Verification items for the finished model (mm, model axes). A direction names the side the tool comes from. Give positions to 0.01 mm unless a question says otherwise; leave off trailing zeros. Loops run counter-clockwise (first coordinate to the right, second up) from the corner with the lowest first, then second, coordinate; pieces in that order, holes last. Notation, with made-up numbers: (61.25, -5.5) -> (69.25, -5.5) arc R19 ccw to (69.25, 12.5) -> close; hole circle Ø8 at (77.25, -15.75). An arc over 180 degrees is marked (long way). Answer in a Markdown table with one row per item. Add a question column.
Q1. Section check A-A on x = 0. Enter the section's corners in (y, z) (3 decimals).
Q2. Section check B-B on z = 2.6. Enter the section's corners in (x, y) (3 decimals).
Q3. Material ranges on probe 1 along Z at (x, y) = (2.25, 0.25); probe 2 along X at (y, z) = (0, 0.1) (3 decimals); probe 3 along Y at (x, z) = (-0.25, 2.4) (3 decimals), recorded low to high.
Q4. Section check D-D on y = 1.5. Enter the section's corners in (x, z), and give its area (3 significant figures).
Q5. Set-up check for faces 1 (the face through (0, 2.625, 2)), 2 (the face through (2, -4.625, 1)), 3 (the face through (3.897, -2, 1)), 4 (the face through (-1, -5, 1)), 5 (the face through (0, 3.625, 1)): record each of +Z, -Z, +X, -X, +Y, -Y from which the full face is reachable in a straight line by a thin tool's end or side.
Q6. Gauge pin test, flat ends, axial feed: P1, Ø0.9, axis at x = 2, z = 2, coming from the -Y side (3 decimals); P2, Ø2.5, axis at x = 0, y = 0, coming from the +Z side; P3, Ø0.8, axis at y = -5.5, z = 1.5, coming from the +X side; P4, Ø3.5, axis at x = 0, y = 0, coming from the +Z side. Record the tip position at first contact, or that the pin passes through.
Q7. Section check C-C on y = -0.5. Enter the section's corners in (x, z), and give its area (3 significant figures).
Q8. Release check for a two-part mould opening along Z. For faces 6 (the face through (-0.3, -1.34, 0.26)), 7 (the face through (2.284, 1.294, 1.514)), 8 (the face through (-2.263, 1.331, 1.514)), 9 (the face through (0, -2, 0)) record: pulls with the +Z half, pulls with the -Z half, needs draft (parallel to the pull), parting line crosses it, or undercut.
```python
from build123d import *

# Parameters (mm, degrees)
SKETCH1_R           = 1.375
BOSS_EXTRUDE1_DEPTH = 3
CUT_EXTRUDE1_DEPTH  = 0.98


with BuildPart() as part:
    # Sketch1 → Boss-Extrude1 (new body)
    with BuildSketch(Plane.XY):
        Polygon((-1, -4.625), (-1, -6.125), (1, -6.125), (1, -4.625), (3.897114317, -4.625), (3.897114317, 0.5), (2.092894726, 3.625), (-2.092894726, 3.625), (-3.897114317, 0.5), (-3.897114317, -4.625), align=None)
        Circle(SKETCH1_R, mode=Mode.SUBTRACT)
    extrude(amount=BOSS_EXTRUDE1_DEPTH)

    # Sketch2 → Cut-Extrude1 (cut, symmetric)
    with BuildSketch(Plane.XY.offset(1.5)):
        Polygon((-1.515544457, -2.625), (1.515544457, -2.625), (3.031088913, 0), (1.515544457, 2.625), (-1.515544457, 2.625), (-3.031088913, 0), align=None)
    extrude(amount=CUT_EXTRUDE1_DEPTH, both=True, mode=Mode.SUBTRACT)


solid = part.part
```
Taken from the geometry:
| question | item | result |
|---|---|---|
| 1 | outline | (-6.125, 0) -> (-1.375, 0) -> (-1.375, 0.52) -> (-2.625, 0.52) -> (-2.625, 2.48) -> (-1.375, 2.48) -> (-1.375, 3) -> (-6.125, 3) -> close; (1.375, 0) -> (3.625, 0) -> (3.625, 3) -> (1.375, 3) -> (1.375, 2.48) -> (2.625, 2.48) -> (2.625, 0.52) -> (1.375, 0.52) -> close |
| 2 | outline | (-3.897, -4.625) -> (-1, -4.625) -> (-1, -6.125) -> (1, -6.125) -> (1, -4.625) -> (3.897, -4.625) -> (3.897, 0.5) -> (2.093, 3.625) -> (-2.093, 3.625) -> (-3.897, 0.5) -> close; hole circle Ø2.75 at (0, 0) |
| 3 | probe 1 | z = 0 to 0.52, 2.48 to 3 |
| 3 | probe 2 | x = -3.897 to -1.375, 1.375 to 3.897 |
| 3 | probe 3 | y = -6.125 to -2.625, 2.625 to 3.625 |
| 4 | outline | (-3.32, 0) -> (3.32, 0) -> (3.32, 3) -> (-3.32, 3) -> close; hole (-2.17, 0.52) -> (2.17, 0.52) -> (2.17, 2.48) -> (-2.17, 2.48) -> close |
| 4 | area | 11.4 mm² |
| 5 | face 1 | none |
| 5 | face 2 | +Z, -Z, +X, -Y |
| 5 | face 3 | +Z, -Z, +X, +Y, -Y |
| 5 | face 4 | +Z, -Z, -X, -Y |
| 5 | face 5 | +Z, -Z, +X, -X, +Y |
| 6 | P1 | stops at y = -4.625 |
| 6 | P2 | passes through |
| 6 | P3 | stops at x = 1 |
| 6 | P4 | stops at z = 3 |
| 7 | outline | (-3.9, 0) -> (-1.28, 0) -> (-1.28, 0.52) -> (-2.74, 0.52) -> (-2.74, 2.48) -> (-1.28, 2.48) -> (-1.28, 3) -> (-3.9, 3) -> close; (1.28, 0) -> (3.9, 0) -> (3.9, 3) -> (1.28, 3) -> (1.28, 2.48) -> (2.74, 2.48) -> (2.74, 0.52) -> (1.28, 0.52) -> close |
| 7 | area | 9.97 mm² |
| 8 | face 6 | needs draft |
| 8 | face 7 | undercut |
| 8 | face 8 | undercut |
| 8 | face 9 | pulls with the -Z half |
